Geometry: final body of the model. Coordinates: model frame, mm. A direction names the side the tool comes from. Round coordinates to 2 decimals unless told otherwise and drop trailing zeros. Order: outer loops, then holes, each group sorted by start corner. A loop starts at its lowest first (then second) coordinate and runs counter-clockwise, first axis right, second up. Notation, with made-up numbers: M -10,31 L 31,31 A31 ccw 31,67 Z; hole C 60,82.25 d1. An arc over 180 degrees is marked long. Return JSON: item names as keys, results as strings. Group by question number.
Q1. Cut plane A-A on x = 3.25. Output: boundary loops of the cut face in (y, z) (3 decimals), and give its area (3 significant figures).
Q2. Ray query, probe 1 along X at (y, z) = (-3, -3.5); probe 2 along Y at (x, z) = (1.5, 6.5); probe 3 along Y at (x, z) = (8.5, 4). Return the intervals inside material, ascending.
Q3. Mould query, pull axis Z, two halves, no side actions, for faces 1 (the face through (6.26, 11.62, 3.66)), 2 (the face through (7.291, 9.378, -3.888)), 3 (the face through (12.7, -3, 10)). Classes: released by +Z, released by -Z, zero draft, split by the parting line, or undercut.
Q4. Access query for faces 4 (the face through (0, 0, 0)), 5 (the face through (2.032, -2.4, 2.4)). Directions: +Z, -Z, +X, -X, +Y, -Y. A direction counts if a zero-diameter tool reaches every point of the face in a straight line with its end or side. Return the directions, or none.
Q5. Contact query for flat-ended pins moving along their axis: pin 1 (1 mm diameter, centred on x = 4, z = -7.5, fed in from -Y); pin 2 (1.5 mm diameter, centred on y = 1, z = -4, fed in from +X); pin 3 (1.5 mm diameter, centred on x = 2, z = -2, fed in from -Y); pin 4 (7.5 mm diameter, centred on y = -2, z = 1, fed in from +X). Output: stop coordinate, or through.
Q6. Cut plane B-B on z = 4. Output: boundary loops of the cut face in (x, y), and give its area (3 significant figures).
Q7. Cut plane C-C on y = 6.5. Output: boundary loops of the cut face in (x, z).
```python
from build123d import *

# Parameters (mm, degrees)
F0_R     = 12.1837068699
F1_DEPTH = 12.7
F2_T     = -2.032
F3_R     = 3.2359024919
F4_DEPTH = 15.24
F6_D     = 6.35
F6_DEPTH = 14.732
F6_TIP   = 1.9077324654


with BuildPart() as f1:
    # F0 (on Right) → F1 (new body)
    with BuildSketch(Plane.YZ):
        Circle(F0_R)
    extrude(amount=F1_DEPTH)

    # F2
    f2_openings = [f1.faces().sort_by_distance(p)[0] for p in [
        (12.7, 0, 0),
    ]]
    offset(amount=F2_T, openings=f2_openings)

    # F3 (on face) → F4 (join)
    with BuildSketch(Plane.YZ.offset(2.032)):
        Circle(F3_R)
    extrude(amount=F4_DEPTH)

    # F6
    with Locations(Plane.YZ.offset(17.272)):
        with Locations((0, 0)):
            Hole(F6_D / 2, depth=F6_DEPTH)
            with Locations((0, 0, -(F6_DEPTH + F6_TIP / 2))):  # 118° drill point
                Cone(0, F6_D / 2, F6_TIP, mode=Mode.SUBTRACT)


solid = f1.part
```
Result sheet:
{
 "1": {"outline": "C 0,0 d24.367; C 0,0 d6.472; hole C 0,0 d20.303; hole C 0,0 d6.35", "area": "144 mm²"},
 "2": {"probe 1": "x = 0 to 2.03", "probe 2": "y = -10.3 to 10.3", "probe 3": "y = -11.51 to -9.33, 9.33 to 11.51"},
 "3": {"face 1": "split by the parting line", "face 2": "undercut", "face 3": "zero draft"},
 "4": {"face 4": "+Z, -Z, -X, +Y, -Y", "face 5": "+X"},
 "5": {"pin 1": "stops at y = -9.97", "pin 2": "stops at x = 2.03", "pin 3": "stops at y = -12.12", "pin 4": "stops at x = 17.27"},
 "6": {"outline": "M 0,-11.51 L 12.7,-11.51 L 12.7,-9.33 L 2.03,-9.33 L 2.03,9.33 L 12.7,9.33 L 12.7,11.51 L 0,11.51 Z", "area": "93.2 mm²"},
 "7": {"outline": "M 0,-10.3 L 12.7,-10.3 L 12.7,-7.8 L 2.03,-7.8 L 2.03,7.8 L 12.7,7.8 L 12.7,10.3 L 0,10.3 Z"}
}
